The model under review builds one solid part; all positions refer to its coordinate system, in mm. Face numbers are marked on the shaded views. A direction names the side the tool comes from. Give positions to 0.01 mm unless a question says otherwise; leave off trailing zeros. Write each loop counter-clockwise with the first axis right and the second up, starting at its lowest first coordinate (ties: lowest second). Pieces come first, ordered by that corner, then holes.
from build123d import *

# Parameters (mm, degrees)
SKETCH_1_W           = 73.4
SKETCH_1_H           = 53.4
SKETCH_1_W_2         = 69.6
SKETCH_1_H_2         = 49.6
EXTRUDE_1_DEPTH      = 17
SKETCH_2_W           = 73.4
SKETCH_2_H           = 53.4
EXTRUDE_2_DEPTH      = 1.5
SKETCH_3_W           = 4.5
SKETCH_3_H           = 4.5
EXTRUDE_3_DEPTH      = 17
SKETCH_9_R           = 3.252691193
EXTRUDE_5_DEPTH      = 2
CHAMFER_1_SIZE       = 0.5
SKETCH_6_OUTSIDE_W   = 93.928
SKETCH_6_OUTSIDE_H   = 73.928
SKETCH_6_OUTSIDE_W_2 = 71.8
SKETCH_6_OUTSIDE_H_2 = 51.8
CUT_EXTRUDE_3_DEPTH  = 5
SKETCH_5_R           = 1.4
CUT_EXTRUDE_2_DEPTH  = 50.010509077
CUT_EXTRUDE_4_REACH  = 68.988
SKETCH_7_W           = 10
SKETCH_7_H           = 6.4
SKETCH_8_R           = 2.5
CUT_EXTRUDE_5_DEPTH  = 2
SKETCH_10_W          = 9.5
SKETCH_10_H          = 6.5
CUT_EXTRUDE_6_DEPTH  = 0.8
CUT_EXTRUDE_7_REACH  = 81.2
SKETCH_11_W          = 8.2
SKETCH_11_H          = 4.5
FILLET_1_R           = 1


with BuildPart() as part:
    # Эскиз1 → Бобышка-Вытянуть1 (new body)
    with BuildSketch(Plane(origin=(0, 0, 0), x_dir=(1, 0, 0), z_dir=(0, 1, 0))):
        Rectangle(SKETCH_1_W, SKETCH_1_H)
        Rectangle(SKETCH_1_W_2, SKETCH_1_H_2, mode=Mode.SUBTRACT)
    extrude(amount=-EXTRUDE_1_DEPTH)

    # Эскиз2 → Бобышка-Вытянуть2 (add)
    with BuildSketch(Plane(origin=(0, 0, 0), x_dir=(1, 0, 0), z_dir=(0, 1, 0))):
        Rectangle(SKETCH_2_W, SKETCH_2_H)
    extrude(amount=EXTRUDE_2_DEPTH)

    # Эскиз3 → Бобышка-Вытянуть3 (add, through all)
    with BuildSketch(Plane(origin=(0, 0, 0), x_dir=(1, 0, 0), z_dir=(0, 1, 0))):
        with Locations((-32.55, 22.55)):
            Rectangle(SKETCH_3_W, SKETCH_3_H)
        with Locations((32.55, 22.55)):
            Rectangle(SKETCH_3_W, SKETCH_3_H)
        with Locations((-32.55, -22.55)):
            Rectangle(SKETCH_3_W, SKETCH_3_H)
        with Locations((32.55, -22.55)):
            Rectangle(SKETCH_3_W, SKETCH_3_H)
    extrude(amount=-EXTRUDE_3_DEPTH)

    # Эскиз9 → Бобышка-Вытянуть5 (add)
    with BuildSketch(Plane(origin=(0, 0, 0), x_dir=(-1, 0, 0), z_dir=(0, 1, 0))):
        with Locations((-33, 23)):
            Circle(SKETCH_9_R)
        with Locations((-33, -23)):
            Circle(SKETCH_9_R)
        with Locations((33, -23)):
            Circle(SKETCH_9_R)
        with Locations((33, 23)):
            Circle(SKETCH_9_R)
    extrude(amount=-EXTRUDE_5_DEPTH)

    # Фаска1
    chamfer_1_edges = [part.edges().sort_by_distance(p)[0] for p in [
        (-36.7, 1.5, 0),
        (0, 1.5, 26.7),
        (36.7, 1.5, 0),
        (0, 1.5, -26.7),
        (-36.7, -7.75, -26.7),
        (36.7, -7.75, -26.7),
        (36.7, -7.75, 26.7),
        (-36.7, -7.75, 26.7),
    ]]
    chamfer(chamfer_1_edges, length=CHAMFER_1_SIZE)

    # Эскиз6 outside → Вырез-Вытянуть3 (cut)
    with BuildSketch(Plane.XZ.offset(17)):
        Rectangle(SKETCH_6_OUTSIDE_W, SKETCH_6_OUTSIDE_H)
        Rectangle(SKETCH_6_OUTSIDE_W_2, SKETCH_6_OUTSIDE_H_2, mode=Mode.SUBTRACT)
    extrude(amount=-CUT_EXTRUDE_3_DEPTH, mode=Mode.SUBTRACT)

    # Эскиз5 → Вырез-Вытянуть2 (cut, through all)
    with BuildSketch(Plane.XZ.offset(17)):
        with Locations(Location((-33, 23, 0), (0, 0, 270))):
            Circle(SKETCH_5_R)
        with Locations(Location((33, 23, 0), (0, 0, 90))):
            Circle(SKETCH_5_R)
        with Locations(Location((33, -23, 0), (0, 0, 270))):
            Circle(SKETCH_5_R)
        with Locations(Location((-33, -23, 0), (0, 0, 90))):
            Circle(SKETCH_5_R)
    extrude(amount=-CUT_EXTRUDE_2_DEPTH, mode=Mode.SUBTRACT)

    # Эскиз7 → Вырез-Вытянуть4 (cut, up to next)
    with BuildSketch(Plane(origin=(0, 0, -26.7), x_dir=(-1, 0, 0), z_dir=(0, 0, -1)), mode=Mode.PRIVATE) as cut_extrude_4_sk1:
        with Locations((-19, -15.2)):
            Rectangle(SKETCH_7_W, SKETCH_7_H)
    cut_extrude_4_tool1 = extrude(cut_extrude_4_sk1.sketch, amount=-CUT_EXTRUDE_4_REACH, mode=Mode.PRIVATE) & part.part
    # Эскиз7 → Вырез-Вытянуть4 (cut, up to next)
    with BuildSketch(Plane(origin=(0, 0, -26.7), x_dir=(-1, 0, 0), z_dir=(0, 0, -1)), mode=Mode.PRIVATE) as cut_extrude_4_sk2:
        with Locations((11.5, -15.2)):
            Rectangle(SKETCH_7_W, SKETCH_7_H)
    cut_extrude_4_tool2 = extrude(cut_extrude_4_sk2.sketch, amount=-CUT_EXTRUDE_4_REACH, mode=Mode.PRIVATE) & part.part
    add(cut_extrude_4_tool1.solids().sort_by_distance((19, -15.2, -26.7))[0], mode=Mode.SUBTRACT)
    add(cut_extrude_4_tool2.solids().sort_by_distance((-11.5, -15.2, -26.7))[0], mode=Mode.SUBTRACT)

    # Эскиз8 → Вырез-Вытянуть5 (cut)
    with BuildSketch(Plane(origin=(0, 1.5, 0), x_dir=(1, 0, 0), z_dir=(0, 1, 0))):
        with Locations(Location((-33, 23, 0), (0, 0, 270))):
            Circle(SKETCH_8_R)
        with Locations(Location((33, 23, 0), (0, 0, 270))):
            Circle(SKETCH_8_R)
        with Locations(Location((33, -23, 0), (0, 0, 270))):
            Circle(SKETCH_8_R)
        with Locations(Location((-33, -23, 0), (0, 0, 270))):
            Circle(SKETCH_8_R)
    extrude(amount=-CUT_EXTRUDE_5_DEPTH, mode=Mode.SUBTRACT)

    # Эскиз10 → Вырез-Вытянуть6 (cut)
    with BuildSketch(Plane.ZY.offset(36.7)):
        with Locations((11.7, -3.25)):
            Rectangle(SKETCH_10_W, SKETCH_10_H)
    extrude(amount=-CUT_EXTRUDE_6_DEPTH, mode=Mode.SUBTRACT)

    # Эскиз11 → Вырез-Вытянуть7 (cut, up to next)
    with BuildSketch(Plane.ZY.offset(35.9), mode=Mode.PRIVATE) as cut_extrude_7_sk1:
        with Locations((11.7, -3.25)):
            Rectangle(SKETCH_11_W, SKETCH_11_H)
    cut_extrude_7_tool1 = extrude(cut_extrude_7_sk1.sketch, amount=-CUT_EXTRUDE_7_REACH, mode=Mode.PRIVATE) & part.part
    add(cut_extrude_7_tool1.solids().sort_by_distance((-35.9, -3.25, 11.7))[0], mode=Mode.SUBTRACT)

    # Скругление1
    # the kernel refuses this fillet: 1 mm, written as the material it adds along each edge
    with BuildSketch(Plane(origin=(-33, 0, -23), x_dir=(-0.9768477562841145, 0, 0.21393564696583717), z_dir=(-0.21393564696583717, 0, -0.9768477562841145))) as fillet_1_piece_1_section:
        with BuildLine():
            CenterArc((3.252691193 + FILLET_1_R, -FILLET_1_R), FILLET_1_R, 90, 90)
            Line((3.252691193, -FILLET_1_R), (3.252691193, 0))
            Line((3.252691193, 0), (3.252691193 + FILLET_1_R, 0))
        make_face()
    fillet_1_piece_1 = revolve(axis=Axis((-33, 0, -23), (0, 1, 0)), revolution_arc=155.58691753, mode=Mode.PRIVATE)
    fillet_1_piece_1 = split(fillet_1_piece_1, bisect_by=Plane(origin=(-34.8, -0.215043292, -19.734246257), z_dir=(1, 0, 0)), keep=Keep.TOP, mode=Mode.PRIVATE)
    add(fillet_1_piece_1)
    with BuildSketch(Plane(origin=(-33, 0, -23), x_dir=(0.20893573542178995, 0, 0.9779293729425228), z_dir=(-0.9779293729425228, 0, 0.20893573542178995))) as fillet_1_piece_2_section:
        with BuildLine():
            CenterArc((3.252691193 + FILLET_1_R, -FILLET_1_R), FILLET_1_R, 90, 90)
            Line((3.252691193, -FILLET_1_R), (3.252691193, 0))
            Line((3.252691193, 0), (3.252691193 + FILLET_1_R, 0))
        make_face()
    fillet_1_piece_2 = revolve(axis=Axis((-33, 0, -23), (0, 1, 0)), revolution_arc=155.58691753, mode=Mode.PRIVATE)
    fillet_1_piece_2 = split(fillet_1_piece_2, bisect_by=Plane(origin=(-31.496865792, -0.203453463, -24.8), z_dir=(0, 0, 1)), keep=Keep.TOP, mode=Mode.PRIVATE)
    add(fillet_1_piece_2)
    with BuildSketch(Plane(origin=(-33, 0, 23), x_dir=(0.21393564696585013, 0, 0.9768477562841116), z_dir=(-0.9768477562841116, 0, 0.21393564696585013))) as fillet_1_piece_3_section:
        with BuildLine():
            CenterArc((3.252691193 + FILLET_1_R, -FILLET_1_R), FILLET_1_R, 90, 90)
            Line((3.252691193, -FILLET_1_R), (3.252691193, 0))
            Line((3.252691193, 0), (3.252691193 + FILLET_1_R, 0))
        make_face()
    fillet_1_piece_3 = revolve(axis=Axis((-33, 0, 23), (0, 1, 0)), revolution_arc=155.58691753, mode=Mode.PRIVATE)
    fillet_1_piece_3 = split(fillet_1_piece_3, bisect_by=Plane(origin=(-29.734246201, -0.215043247, 24.8), z_dir=(0, 0, -1)), keep=Keep.TOP, mode=Mode.PRIVATE)
    add(fillet_1_piece_3)
    with BuildSketch(Plane(origin=(-33, 0, 23), x_dir=(0.9779293729425067, 0, -0.20893573542186514), z_dir=(0.20893573542186514, 0, 0.9779293729425067))) as fillet_1_piece_4_section:
        with BuildLine():
            CenterArc((3.252691193 + FILLET_1_R, -FILLET_1_R), FILLET_1_R, 90, 90)
            Line((3.252691193, -FILLET_1_R), (3.252691193, 0))
            Line((3.252691193, 0), (3.252691193 + FILLET_1_R, 0))
        make_face()
    fillet_1_piece_4 = revolve(axis=Axis((-33, 0, 23), (0, 1, 0)), revolution_arc=155.58691753, mode=Mode.PRIVATE)
    fillet_1_piece_4 = split(fillet_1_piece_4, bisect_by=Plane(origin=(-34.8, -0.203453257, 21.496866097), z_dir=(1, 0, 0)), keep=Keep.TOP, mode=Mode.PRIVATE)
    add(fillet_1_piece_4)
    with BuildSketch(Plane(origin=(33, 0, 23), x_dir=(0.9768477562841055, 0, -0.21393564696587863), z_dir=(0.21393564696587863, 0, 0.9768477562841055))) as fillet_1_piece_5_section:
        with BuildLine():
            CenterArc((3.252691193 + FILLET_1_R, -FILLET_1_R), FILLET_1_R, 90, 90)
            Line((3.252691193, -FILLET_1_R), (3.252691193, 0))
            Line((3.252691193, 0), (3.252691193 + FILLET_1_R, 0))
        make_face()
    fillet_1_piece_5 = revolve(axis=Axis((33, 0, 23), (0, 1, 0)), revolution_arc=155.58691753, mode=Mode.PRIVATE)
    fillet_1_piece_5 = split(fillet_1_piece_5, bisect_by=Plane(origin=(34.8, -0.215043292, 19.734246257), z_dir=(-1, 0, 0)), keep=Keep.TOP, mode=Mode.PRIVATE)
    add(fillet_1_piece_5)
    with BuildSketch(Plane(origin=(33, 0, 23), x_dir=(-0.20893573542180963, 0, -0.9779293729425186), z_dir=(0.9779293729425186, 0, -0.20893573542180963))) as fillet_1_piece_6_section:
        with BuildLine():
            CenterArc((3.252691193 + FILLET_1_R, -FILLET_1_R), FILLET_1_R, 90, 90)
            Line((3.252691193, -FILLET_1_R), (3.252691193, 0))
            Line((3.252691193, 0), (3.252691193 + FILLET_1_R, 0))
        make_face()
    fillet_1_piece_6 = revolve(axis=Axis((33, 0, 23), (0, 1, 0)), revolution_arc=155.58691753, mode=Mode.PRIVATE)
    fillet_1_piece_6 = split(fillet_1_piece_6, bisect_by=Plane(origin=(31.496865792, -0.203453463, 24.8), z_dir=(0, 0, -1)), keep=Keep.TOP, mode=Mode.PRIVATE)
    add(fillet_1_piece_6)
    with BuildSketch(Plane(origin=(33, 0, -23), x_dir=(-0.2139356469658719, 0, -0.9768477562841068), z_dir=(0.9768477562841068, 0, -0.2139356469658719))) as fillet_1_piece_7_section:
        with BuildLine():
            CenterArc((3.252691193 + FILLET_1_R, -FILLET_1_R), FILLET_1_R, 90, 90)
            Line((3.252691193, -FILLET_1_R), (3.252691193, 0))
            Line((3.252691193, 0), (3.252691193 + FILLET_1_R, 0))
        make_face()
    fillet_1_piece_7 = revolve(axis=Axis((33, 0, -23), (0, 1, 0)), revolution_arc=155.58691753, mode=Mode.PRIVATE)
    fillet_1_piece_7 = split(fillet_1_piece_7, bisect_by=Plane(origin=(29.734246201, -0.215043247, -24.8), z_dir=(0, 0, 1)), keep=Keep.TOP, mode=Mode.PRIVATE)
    add(fillet_1_piece_7)
    with BuildSketch(Plane(origin=(33, 0, -23), x_dir=(-0.9779293729425086, 0, 0.20893573542185656), z_dir=(-0.20893573542185656, 0, -0.9779293729425086))) as fillet_1_piece_8_section:
        with BuildLine():
            CenterArc((3.252691193 + FILLET_1_R, -FILLET_1_R), FILLET_1_R, 90, 90)
            Line((3.252691193, -FILLET_1_R), (3.252691193, 0))
            Line((3.252691193, 0), (3.252691193 + FILLET_1_R, 0))
        make_face()
    fillet_1_piece_8 = revolve(axis=Axis((33, 0, -23), (0, 1, 0)), revolution_arc=155.58691753, mode=Mode.PRIVATE)
    fillet_1_piece_8 = split(fillet_1_piece_8, bisect_by=Plane(origin=(34.8, -0.203453257, -21.496866097), z_dir=(-1, 0, 0)), keep=Keep.TOP, mode=Mode.PRIVATE)
    add(fillet_1_piece_8)


solid = part.part
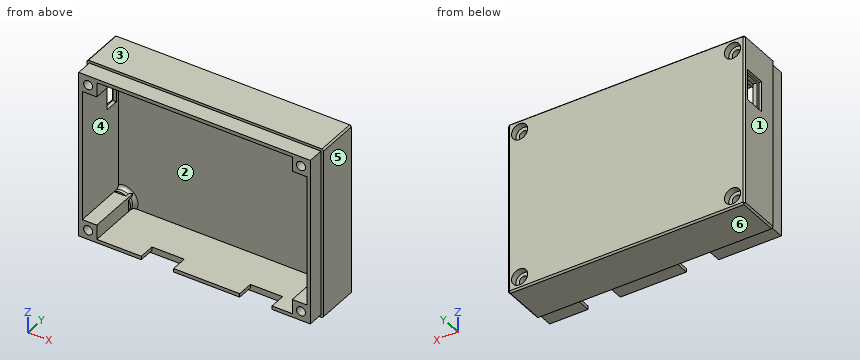
1) Tool access review of the marked faces 1 and 2: name each direction out of +Z, -Z, +X, -X, +Y, -Y from which nothing blocks a thin tool from reaching the whole face with its end or side.
2) Consider section B-B, the plane x = -26.5. Give the boundary of the cut face in (y, z), then the cut area to 3 significant figures.
3) Consider section C-C, the plane x = 33. State how many separate pieces and enclosed holes the cut face has, then the cut area to 3 significant figures.
4) The part is to be moulded in two halves that separate along Z. For the marked faces 3, 4, 5 and 6, say which applies: +Z half, -Z half, draft (parallel to the pull), parting line (faces both ways), or undercut.
5) Consider section A-A, the plane z = -14.5. Give the boundary of the cut face in (x, y), then the cut area to 3 significant figures.
6) Insertion check: pin 1 (3 mm diameter, centred on y = -4.5, z = 10.5, fed in from -X); pin 2 (10 mm diameter, centred on x = 16.5, z = 18.5, fed in from -Y); pin 3 (1.7 mm diameter, centred on x = 33, z = 23, fed in from -Y); pin 4 (0.5 mm diameter, centred on y = -15, z = -25.5, fed in from +X). Each pin has a flat end and moves straight along its axis. Give the tip position at first contact, or say it passes through.
7) To check wall thickness, follow probe 1 along X at (y, z) = (-13.5, 23); probe 2 along X at (y, z) = (-11.25, 23); probe 3 along X at (y, z) = (-6.5, -11). State the ranges of each line that lie inside material, in increasing order.
Answer block:
1. face 1: +Z, -Z, -X, +Y, -Y
1. face 2: -Y
2. outline: (-17, -25.9) - (-12, -25.9) - (-12, -26.7) - (1, -26.7) - (1.5, -26.2) - (1.5, 26.2) - (1, 26.7) - (-12, 26.7) - (-12, 25.9) - (-17, 25.9) - (-17, 24.8) - (0, 24.8) - (0, -24.8) - (-17, -24.8) - close
2. area: 136 mm2
3. separate pieces: 3
3. enclosed holes: 0
3. area: 180 mm2
4. face 3: +Z half
4. face 4: undercut
4. face 5: draft
4. face 6: -Z half
5. outline: (-36.7, -12) - (-35.9, -12) - (-35.9, -17) - (-34.8, -17) - (-34.8, 0) - (34.8, 0) - (34.8, -17) - (35.9, -17) - (35.9, -12) - (36.7, -12) - (36.7, 1) - (36.2, 1.5) - (-36.2, 1.5) - (-36.7, 1) - close
5. area: 166 mm2
6. pin 1: stops at x = -35.9
6. pin 2: stops at y = 0
6. pin 3: passes through
6. pin 4: stops at x = 35.9
7. probe 1: x = -35.9 to -34.4, -31.6 to -30.3, 30.3 to 31.6, 34.4 to 35.9
7. probe 2: x = -36.7 to -34.4, -31.6 to -30.3, 30.3 to 31.6, 34.4 to 36.7
7. probe 3: x = -36.7 to -34.8, 34.8 to 36.7
